Here's how the part is built. I have some questions about the finished solid (model axes, mm). A direction names the side the tool comes from. Give positions to 0.01 mm unless a question says otherwise; leave off trailing zeros. Loops run counter-clockwise (first coordinate to the right, second up) from the corner with the lowest first, then second, coordinate; pieces in that order, holes last. Notation, with made-up numbers: (31, 75) -> (38, 75) arc R17 ccw to (38, 92) -> close; hole circle Ø9 at (-8.75, 41). An arc over 180 degrees is marked (long way). Answer in a Markdown table with one row per item. Add a question column.
Item 1: If we section it at C-C (z = 0): Write out the boundary of the cut face in (x, y).
Item 2: If we section it at B-B (y = -20): Write out the boundary of the cut face in (x, z), then the cut area to 3 significant figures.
Item 3: If I drill on line 1 (Z direction, x = 0, y = 6); line 2 (Y direction, x = -27.5, z = -42); line 3 (Y direction, x = -1.5, z = -57), over which ranges is the centre line in solid material (lowest first)?
Item 4: If we section it at A-A (x = 0): Write out the boundary of the cut face in (y, z), then the cut area to 3 significant figures.
Item 5: If we section it at D-D (z = -53): Write out the boundary of the cut face in (x, y).
Item 6: For P1, Ø2, axis at x = -8.5, y = -16, coming from the +Z side; P2, Ø4.5, axis at y = -21, z = -53, coming from the -X side; P3, Ø6, axis at y = -17.5, z = 16.5, coming from the +X side (3 decimals), each with a flat end and sliding along its axis, tell me the tip position at first contact or that it passes through.
Item 7: Which directions (+Z, -Z, +X, -X, +Y, -Y) give clear straight access to the entire face, cutting with the end or side of a thin tool? Please do faces 4 (the face through (-10, -20, -51)), 5 (the face through (4.77, -7.1, -52.3)), 6 (the face through (-16, 10, 1)), 7 (the face through (10, -20, -51)), 8 (the face through (-38.903, -20.105, 34.008)).
Item 8: We'd pull the mould along X, two halves only. Please class faces 1 (the face through (-2.17, 5.07, 9.76)), 2 (the face through (48.903, -20.105, 16.687)), 3 (the face through (-48.903, -20.105, 16.687)): released by +X, released by -X, zero draft, split by the parting line, or undercut.
Autodesk Inventor part; units mm, degrees
ref_plane "YZ Plane" through (0, 0, 0) normal (1, 0, 0) x (0, 1, 0)
ref_plane "XZ Plane" through (0, 0, 0) normal (0, 1, 0) x (-1, 0, 0)
ref_plane "XY Plane" through (0, 0, 0) normal (0, 0, 1) x (1, 0, 0)
sketch "Sketch1" plane through (0, 0, 0) normal (0, 1, 0) x (-1, 0, 0)
  circle A0 centre (0, 0) radius 76.2
  dimension "d0" = 152.4
extrude "Extrusion1" add sketch "Sketch1" along normal blind 10
sketch "Sketch2" plane through (0, 0, 0) normal (0, -1, 0) x (1, 0, 0)
  circle A0 centre (0, -50.8) radius 5
  line L0 (0, 0) -> (0, -50.8)
  dimension "d3" = 50.8
  dimension "d4" = 10
extrude "Extrusion2" add sketch "Sketch2" along normal blind 20
pattern_circular "Circular Pattern1" count 3 over 360 about axis through (0, -10, 0) along (0, 1, 0) of "Extrusion2"
sketch "Sketch4" plane through (0, 10, 0) normal (0, 1, 0) x (1, 0, 0)
  circle A0 centre (0, 0) radius 10
  dimension "d12" = 20
extrude "Extrusion3" cut sketch "Sketch4" against normal up to surface (10 mm away)
sketch "Sketch5" plane through (0, 0, 0) normal (1, 0, 0) x (0, 1, 0)
  line L0 (-20, -45.8) -> (-20, -55.8)
  circle A0 centre (-20, -50.8) radius 7.5
  point P0 (0, 0)
  dimension "d15" = 15
extrude "Extrusion4" add sketch "Sketch5" along normal mid plane 20
pattern_circular "Circular Pattern2" count 3 over 360 about axis through (0, 0, 0) along (0, 1, 0) of "Extrusion4"
properties part number "pll-base"
Recorded:
| question | item | result |
|---|---|---|
| 1 | outline | (-76.2, 0) -> (-10, 0) -> (-10, 10) -> (-76.2, 10) -> close; (10, 0) -> (76.2, 0) -> (76.2, 10) -> (10, 10) -> close |
| 2 | outline | (-55.49, 20.49) -> (-42.5, 12.99) -> (-32.5, 30.31) -> (-45.49, 37.81) -> close; (-10, -58.3) -> (10, -58.3) -> (10, -43.3) -> (-10, -43.3) -> close; (32.5, 30.31) -> (42.5, 12.99) -> (55.49, 20.49) -> (45.49, 37.81) -> close |
| 2 | area | 900 mm^2 |
| 3 | line 1 | z = -76.2 to -10, 10 to 76.2 |
| 3 | line 2 | y = 0 to 10 |
| 3 | line 3 | y = -24.22 to -15.78, 0 to 10 |
| 4 | outline | (-14.41, -55.8) -> (0, -55.8) -> (0, -76.2) -> (10, -76.2) -> (10, -10) -> (0, -10) -> (0, -45.8) -> (-14.41, -45.8) arc R7.5 ccw (long way) to start; (0, 10) -> (10, 10) -> (10, 76.2) -> (0, 76.2) -> close |
| 4 | area | 1,630 mm^2 |
| 5 | outline | (-54.75, 0) -> (-4.49, 0) -> (-4.49, -12.83) -> (-10, -12.83) -> (-10, -27.17) -> (10, -27.17) -> (10, -12.83) -> (4.49, -12.83) -> (4.49, 0) -> (54.75, 0) -> (54.75, 10) -> (-54.75, 10) -> close |
| 6 | P1 | stops at z = -43.93 |
| 6 | P2 | stops at x = -10 |
| 6 | P3 | stops at x = 53.775 |
| 7 | face 4 | +Z, -Z, -X, -Y |
| 7 | face 5 | none |
| 7 | face 6 | +Z, -Z, +X, -X, +Y |
| 7 | face 7 | +Z, -Z, +X, -Y |
| 7 | face 8 | +Z, -Y |
| 8 | face 1 | undercut |
| 8 | face 2 | released by +X |
| 8 | face 3 | released by -X |
